```python
from build123d import *

# Parameters (mm, degrees)
CYLINDER001_R          = 1.8
CYLINDER001_DEPTH      = 100
CYLINDER_R             = 1.8
CYLINDER_DEPTH         = 100
BOX001_W               = 25
BOX001_H               = 60
BOX001_DEPTH           = 25
BOX001_PLACEMENT_ANGLE = 30.25
BOX_W                  = 65
BOX_H                  = 44
BOX_DEPTH              = 2


with BuildPart() as zylinder001:
    # Cylinder001 → Cylinder001 (new body)
    with BuildSketch(Plane(origin=(29.5, 5.5, -6), x_dir=(1, 0, 0), z_dir=(0, 0, 1))):
        Circle(CYLINDER001_R)
    extrude(amount=CYLINDER001_DEPTH)


with BuildPart() as zylinder:
    # Cylinder → Cylinder (new body)
    with BuildSketch(Plane(origin=(29.5, 38.5, -6), x_dir=(1, 0, 0), z_dir=(0, 0, 1))):
        Circle(CYLINDER_R)
    extrude(amount=CYLINDER_DEPTH)


with BuildPart() as obj1:
    # Box001 → Box001 (new body)
    with BuildSketch(Plane.XY):
        with Locations((12.5, 30)):
            Rectangle(BOX001_W, BOX001_H)
    extrude(amount=BOX001_DEPTH)


with BuildPart() as obj1_1:
    # Box001 placement: moved
    add(obj1.part.moved(Location((8, -18, 0))).rotate(Axis((8, -18, 0), (0, 0, 1)), BOX001_PLACEMENT_ANGLE))


with BuildPart() as cut008:
    # Box → Box (new body)
    with BuildSketch(Plane.XY):
        with Locations((32.5, 22)):
            Rectangle(BOX_W, BOX_H)
    extrude(amount=BOX_DEPTH)

    # Cut003: cut obj1
    add(obj1_1.part, mode=Mode.SUBTRACT)


with BuildPart() as cut008_1:
    # Cut003 placement: moved
    add(cut008.part.moved(Location((0, 0, 50))))

    # Cut007: cut Zylinder
    add(zylinder.part, mode=Mode.SUBTRACT)

    # Cut008: cut Zylinder001
    add(zylinder001.part, mode=Mode.SUBTRACT)


solid = cut008_1.part
```
Here's how the part is built. I have some questions about the finished solid (model axes, mm). Round coordinates to 2 decimals unless told otherwise and drop trailing zeros. Order: outer loops, then holes, each group sorted by start corner. A loop starts at its lowest first (then second) coordinate and runs counter-clockwise, first axis right, second up. Notation, with made-up numbers: (24.25, 9.25) -> (35.25, 9.25) arc R33 cw to (35.25, 43.25) -> close; hole circle Ø7 at (74, -7). An arc over 180 degrees is marked (long way). Use a Markdown table: item, result. Add a question column.
(1) Suppose I cut it at D-D, the plane y = 6.5. Please give me the cut outline in (x, z), and give its area (3 significant figures).
(2) If we mould it in two halves opening along Y, with no side actions, what happens to faces 1 (the face through (40, 22, 50)), 2 (the face through (31.163, 4.811, 50.986)), 3 (the face through (45, 0, 51))? For each: released by +Y, released by -Y, zero draft, split by the parting line, or undercut.
(3) Suppose I cut it at B-B, the plane y = 38.5. Please give me the cut outline in (x, z).
(4) Suppose I cut it at C-C, the plane z = 51.6. Please give me the cut outline in (x, y).
(5) I need wall thicknesses on line 1 along Y through (x, z) = (29.5, 50.8); line 2 along X through (y, z) = (5, 50.25); line 3 along X through (y, z) = (38.5, 51.5). Which ranges of each line are inside material? Lowest first, please.
(6) Suppose I cut it at A-A, the plane x = 29.5. Please give me the cut outline in (y, z), and give its area (3 significant figures).
Verdict:
| question | item | result |
|---|---|---|
| 1 | outline | (22.65, 50) -> (28, 50) -> (28, 52) -> (22.65, 52) -> close; (31, 50) -> (65, 50) -> (65, 52) -> (31, 52) -> close |
| 1 | area | 78.7 mm2 |
| 2 | face 1 | zero draft |
| 2 | face 2 | undercut |
| 2 | face 3 | released by -Y |
| 3 | outline | (3.99, 50) -> (27.7, 50) -> (27.7, 52) -> (3.99, 52) -> close; (31.3, 50) -> (65, 50) -> (65, 52) -> (31.3, 52) -> close |
| 4 | outline | (0.78, 44) -> (26.44, 0) -> (65, 0) -> (65, 44) -> close; hole circle Ø3.6 at (29.5, 5.5); hole circle Ø3.6 at (29.5, 38.5) |
| 5 | line 1 | 0 to 3.7, 7.3 to 36.7, 40.3 to 44 |
| 5 | line 2 | 23.53 to 27.77, 31.23 to 65 |
| 5 | line 3 | 3.99 to 27.7, 31.3 to 65 |
| 6 | outline | (0, 50) -> (3.7, 50) -> (3.7, 52) -> (0, 52) -> close; (7.3, 50) -> (36.7, 50) -> (36.7, 52) -> (7.3, 52) -> close; (40.3, 50) -> (44, 50) -> (44, 52) -> (40.3, 52) -> close |
| 6 | area | 73.6 mm2 |
